Verification items for the finished model (mm, model axes). Face numbers are marked on the shaded views. A direction names the side the tool comes from. Give positions to 0.01 mm unless a question says otherwise; leave off trailing zeros. Loops run counter-clockwise (first coordinate to the right, second up) from the corner with the lowest first, then second, coordinate; pieces in that order, holes last. Notation, with made-up numbers: M 32.25,9 L 62.25,9 A18 cw 62.25,32 Z; hole C 30.5,56.25 d4. An arc over 180 degrees is marked long. Use a Markdown table: item, result.
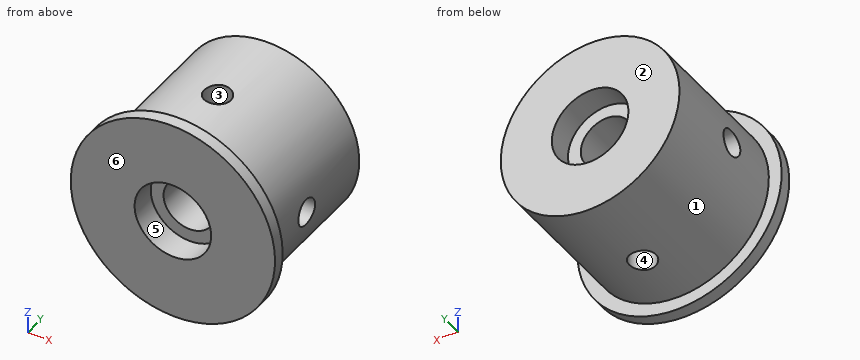
from build123d import *

# Parameters (mm, degrees)
CUT_EXTRUDE1_REACH      = 31.471
CUT_EXTRUDE1_END_RADIUS = 11.1125
CUT_EXTRUDE1_START      = -5.5
SKETCH2_R               = 1.65
CIRPATTERN1_COUNT       = 4


with BuildPart() as part:
    # Sketch1 → Revolve1 (revolve)
    with BuildSketch(Plane(origin=(0, 0, 0), x_dir=(0, 0, -1), z_dir=(1, 0, 0)), mode=Mode.PRIVATE) as revolve1_sk:
        Polygon((-3.175, 0), (-4.7625, 0), (-4.7625, -3.175), (-12.7, -3.175), (-12.7, -1.675), (-11.1125, -1.675), (-11.1125, 15.875), (-4.7625, 15.875), (-4.7625, 12.7), (-3.175, 12.7), align=None)
    revolve(revolve1_sk.sketch.rotate(Axis((0, -1000, 0), (0, 1, 0)), 180), axis=Axis((0, -1000, 0), (0, 1, 0)))

    # Cut-Extrude1: up to this cylinder (the profile starts inside it)
    cut_extrude1_end = Plane(origin=(0, 5.575, 0), z_dir=(0, -1, 0)) * Cylinder(CUT_EXTRUDE1_END_RADIUS, 86.167, mode=Mode.PRIVATE)
    # Sketch2 → Cut-Extrude1 (cut, up to the surface)
    with BuildSketch(Plane(origin=(0, 0, 0), x_dir=(0, 0, -1), z_dir=(1, 0, 0)).offset(CUT_EXTRUDE1_START), mode=Mode.PRIVATE) as cut_extrude1_sk1:
        with Locations((0, 5.575)):
            Circle(SKETCH2_R)
    cut_extrude1_tool1 = extrude(cut_extrude1_sk1.sketch, amount=-CUT_EXTRUDE1_REACH, mode=Mode.PRIVATE) & cut_extrude1_end
    cut_extrude1 = cut_extrude1_tool1.solids().sort_by_distance((-5.5, 5.575, 0))[0]
    add(cut_extrude1, mode=Mode.SUBTRACT)

    # CirPattern1: Cut-Extrude1 ×4 about axis
    cirpattern1_axis = Axis((0, 0, 0), (0, 1, 0))
    for i in range(1, CIRPATTERN1_COUNT):
        add(cut_extrude1.rotate(cirpattern1_axis, i * 360 / CIRPATTERN1_COUNT), mode=Mode.SUBTRACT)


solid = part.part
(1) Gauge pin test, flat ends, axial feed: P1, Ø5, axis at x = -1.5, z = -2, coming from the -Y side (3 decimals); P2, Ø2.5, axis at x = 0, y = 6.5, coming from the -Z side; P3, Ø1.5, axis at y = 5, z = 7, coming from the -X side; P4, Ø2.5, axis at y = 5.575, z = 0, coming from the -X side. Record the tip position at first contact, or that the pin passes through.
Results below:
| item | result |
|---|---|
| P1 | y = -3.175 |
| P2 | z = -11.11 |
| P3 | x = -9.19 |
| P4 | x = -5.5 |
(2) Material ranges on line 1 (Y direction, x = -8.2, z = 0) (3 decimals); line 2 (X direction, y = -1.35, z = 0); line 3 (Y direction, x = 7.75, z = 8.75) (3 decimals), recorded low to high.
Results below:
| item | result |
|---|---|
| line 1 | -3.175 to 3.925, 7.225 to 15.875 |
| line 2 | -11.11 to -4.76, 4.76 to 11.11 |
| line 3 | -3.175 to -1.675 |
(3) Set-up check for the marked faces 1, 2 and 3: record each of +Z, -Z, +X, -X, +Y, -Y from which the full face is reachable in a straight line by a thin tool's end or side.
Results below:
| item | result |
|---|---|
| face 1 | +Y |
| face 2 | +Z, -Z, +X, -X, +Y |
| face 3 | +Z |
(4) Cross-section at A-A on x = 0. Record the cut outline in (y, z) (1 decimal), then the cut area to 3 significant figures.
Results below:
| item | result |
|---|---|
| outline | M -3.2,-12.7 L -1.7,-12.7 L -1.7,-11.1 L 3.9,-11.1 L 3.9,-5.5 L 7.2,-5.5 L 7.2,-11.1 L 15.9,-11.1 L 15.9,-4.8 L 12.7,-4.8 L 12.7,-3.2 L 0,-3.2 L 0,-4.8 L -3.2,-4.8 Z; M -3.2,4.8 L 0,4.8 L 0,3.2 L 12.7,3.2 L 12.7,4.8 L 15.9,4.8 L 15.9,11.1 L 7.2,11.1 L 7.2,5.5 L 3.9,5.5 L 3.9,11.1 L -1.7,11.1 L -1.7,12.7 L -3.2,12.7 Z |
| area | 250 mm^2 |
(5) Cross-section at D-D on x = 9. Record the cut outline in (y, z) (3 decimals), then the cut area to 3 significant figures.
Results below:
| item | result |
|---|---|
| outline | M -3.175,-8.96 L -1.675,-8.96 L -1.675,-6.518 L 15.875,-6.518 L 15.875,6.518 L -1.675,6.518 L -1.675,8.96 L -3.175,8.96 Z; hole C 5.575,0 d3.3 |
| area | 247 mm^2 |
(6) Cross-section at B-B on z = 0. Record the cut outline in (x, y) (1 decimal), then the cut area to 3 significant figures.
Results below:
| item | result |
|---|---|
| outline | M -12.7,-3.2 L -4.8,-3.2 L -4.8,0 L -3.2,0 L -3.2,12.7 L -4.8,12.7 L -4.8,15.9 L -11.1,15.9 L -11.1,7.2 L -5.5,7.2 L -5.5,3.9 L -11.1,3.9 L -11.1,-1.7 L -12.7,-1.7 Z; M 3.2,0 L 4.8,0 L 4.8,-3.2 L 12.7,-3.2 L 12.7,-1.7 L 11.1,-1.7 L 11.1,3.9 L 5.5,3.9 L 5.5,7.2 L 11.1,7.2 L 11.1,15.9 L 4.8,15.9 L 4.8,12.7 L 3.2,12.7 Z |
| area | 250 mm^2 |
(7) Draft check along Y on the marked faces 4, 5 and 6. Enter one of: +Y half, -Y half, draft (parallel to the pull), parting line (faces both ways), or undercut.
Results below:
| item | result |
|---|---|
| face 4 | undercut |
| face 5 | draft |
| face 6 | -Y half |
